from build123d import *

# Parameters (mm, degrees)
F0_R     = 7.5
F1_DEPTH = 13
F2_R     = 3.05
F3_DEPTH = 12
F5_R     = 3.05
F6_DEPTH = 10
F8_DEPTH = 5
F9_R     = 2


with BuildPart() as f1:
    # F0 (on Top) → F1 (new body)
    with BuildSketch(Plane.XY):
        Circle(F0_R)
    extrude(amount=F1_DEPTH)

    # F2 (on face) → F3 (cut)
    with BuildSketch(Plane.XY.offset(13)):
        Circle(F2_R)
    extrude(amount=-F3_DEPTH, mode=Mode.SUBTRACT)

    # F5 (on face) → F6 (cut)
    with BuildSketch(Plane.XY.offset(13)):
        Polygon((5.8257949863, -0.2518851143), (3.1310364009, 4.9193438983), (-2.6947585854, 5.1712290125), (-5.8257949863, 0.2518851143), (-3.1310364009, -4.9193438983), (2.6947585854, -5.1712290125), align=None)
        Circle(F5_R, mode=Mode.SUBTRACT)
    extrude(amount=-F6_DEPTH, mode=Mode.SUBTRACT)

    # F7 (on face) → F8 (cut)
    with BuildSketch(Plane.XY.offset(13)):
        with BuildLine():
            Line((-3.1310364009, -4.9193438983), (-5.8257949863, 0.2518851143))
            Line((-5.8257949863, 0.2518851143), (-5.8257949863, -4.7233582097))
            ThreePointArc((-5.8257949863, -4.7233582097), (0, -7.5), (5.8257949863, -4.7233582097))
            Line((5.8257949863, -4.7233582097), (5.8257949863, -0.2518851143))
            Line((5.8257949863, -0.2518851143), (2.6947585854, -5.1712290125))
            Line((2.6947585854, -5.1712290125), (-3.1310364009, -4.9193438983))
        make_face()
    extrude(amount=-F8_DEPTH, mode=Mode.SUBTRACT)

    # F9
    f9_edges = [f1.edges().sort_by_distance(p)[0] for p in [
        (-7.5, 0, 0),
    ]]
    fillet(f9_edges, radius=F9_R)


solid = f1.part
Model file for the job. Use its own axes, mm. A direction names the side the tool comes from. Round coordinates to 2 decimals unless told otherwise and drop trailing zeros. Order: outer loops, then holes, each group sorted by start corner. A loop starts at its lowest first (then second) coordinate and runs counter-clockwise, first axis right, second up. Notation, with made-up numbers: M 85,10.5 L 122,10.5 A18 ccw 122,17.5 Z; hole C -6.5,-31 d3. An arc over 180 degrees is marked long. Write each question's results on one line, items separated by ' | '. Start each with the question number.
(1) Saw through at D-D, the plane z = 10. Give the cut face in (x, y).
(2) Two-plate mould, pull along X, no slides. Class faces 1 (the face through (-0.976, 7.436, 7.423)), 2 (the face through (0, 0, 0)), 3 (the face through (-3.047, 0.134, 2.014)), 4 (the face through (-4.497, -2.298, 5.535)): pulls with the +X half, pulls with the -X half, needs draft (parallel to the pull), parting line crosses it, or undercut.
(3) Saw through at A-A, the plane z = 5. Give the cut face in (x, y), then the cut area to 3 significant figures.
(4) Which spindle directions (+Z, -Z, +X, -X, +Y, -Y) get a long thin tool onto all of the face, cutting with end or side? Do faces 5 (the face through (-4.238, 2.746, 8.07)), 6 (the face through (5.826, -3, 11)), 7 (the face through (0.5, 5.5, 13)). Say none if no direction does.
(5) Drop flat-ended pins along their axis: pin 1 (3 mm diameter, centred on x = -2.5, y = 1.5, fed in from +Z); pin 2 (5.5 mm diameter, centred on x = 0, y = 0, fed in from +Z); pin 3 (3 mm diameter, centred on y = -3.5, z = 6.5, fed in from -X). Give the stop position or say it passes through.
(6) Saw through at C-C, the plane x = 0. Give the cut face in (y, z), then the cut area to 3 significant figures.
(7) Probe probe 1 along Y at (x, z) = (0, 1.9); probe 2 along Z at (x, y) = (-3.5, -4); probe 3 along Y at (x, z) = (0, 1.55). List the from-to ranges inside material, lowest first. Write a range as from..to.
(8) Saw through at B-B, the plane y = 0. Give the cut face in (x, z).
Established:
1) outline: M -5.83,-4.72 L -5.83,0.25 L -2.69,5.17 L 3.13,4.92 L 5.83,-0.25 L 5.83,-4.72 A7.5 ccw long Z
2) face 1: parting line crosses it | face 2: needs draft | face 3: undercut | face 4: undercut
3) outline: C 0,0 d15; hole M -5.83,0.25 L -3.13,-4.92 L 2.69,-5.17 L 5.83,-0.25 L 3.13,4.92 L -2.69,5.17 Z | area: 88.4 mm^2
4) face 5: +Z | face 6: +Z, -Y | face 7: +Z, +X, -X, +Y, -Y
5) pin 1: stops at z = 3 | pin 2: stops at z = 1 | pin 3: stops at x = -7.23
6) outline: M -7.5,2 A2 ccw -5.5,0 L 5.5,0 A2 ccw 7.5,2 L 7.5,13 L 5.05,13 L 5.05,3 L 3.05,3 L 3.05,1 L -3.05,1 L -3.05,3 L -5.05,3 L -5.05,8 L -7.5,8 Z | area: 67.8 mm^2
7) probe 1: y = -7.5..-3.05, 3.05..7.5 | probe 2: z = 0..3 | probe 3: y = -7.45..-3.05, 3.05..7.45
8) outline: M -7.5,2 A2 ccw -5.5,0 L 5.5,0 A2 ccw 7.5,2 L 7.5,13 L 5.69,13 L 5.69,3 L 3.05,3 L 3.05,1 L -3.05,1 L -3.05,3 L -5.69,3 L -5.69,8 L -5.83,8 L -5.83,13 L -7.5,13 Z
